Check sheet for the modelled part. Datum: model origin and axes. Units: mm. Face numbers are marked on the shaded views. A direction names the side the tool comes from. Coordinates: 2 decimals unless noted, no trailing zeros. Loops run counter-clockwise (first coordinate to the right, second up) from the corner with the lowest first, then second, coordinate; pieces in that order, holes last.
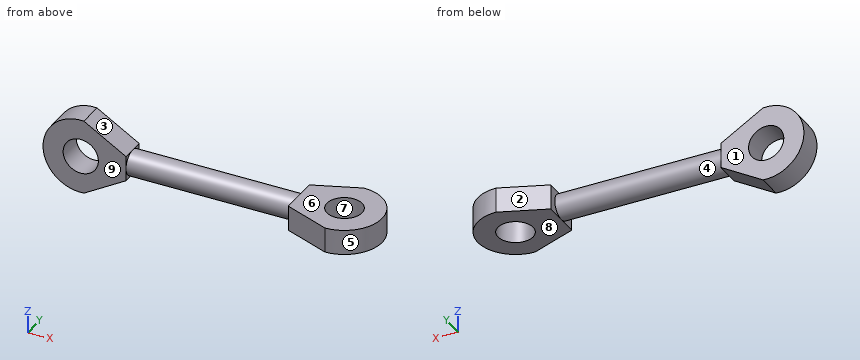
```python
from build123d import *

# Parameters (mm, degrees)
BOSS_EXTRUDE2_DEPTH = 2.5
SKETCH4_R           = 2.5
BOSS_EXTRUDE3_DEPTH = 33.000000000000014
SKETCH8_R           = 3.5000000000000004
BOSS_EXTRUDE4_DEPTH = 2.5


with BuildPart() as part:
    # Sketch1 → Boss-Extrude2 (new, symmetric)
    with BuildSketch(Plane.XY):
        with BuildLine():
            ThreePointArc((7.5, -3.5307e-13), (5.303300858899232, 5.303300858898982), (1.36e-15, 7.500000000000001))
            Line((0, 7.5), (-9.088423691387959, 4))
            Line((-9.088423691387959, 4), (-9.088423691387959, 0))
            Line((-9.088423691387959, 0), (-3.5, 0))
            ThreePointArc((-3.5, 4.3e-16), (2.1e-16, 3.5), (3.5, 0))
            Line((3.5, 0), (7.5, 0))
        make_face()
        with BuildLine():
            ThreePointArc((0, -7.499999999999999), (5.303300858898981, -5.303300858899231), (7.5, -3.5307e-13))
            Line((7.5, 0), (3.5, 0))
            ThreePointArc((3.5, -8.6e-16), (-6.4e-16, -3.5), (-3.5, 4.3e-16))
            Line((-3.5, 0), (-9.088423691387959, 0))
            Line((-9.088423691387959, 0), (-9.088423691387959, -4))
            Line((-9.088423691387959, -4), (0, -7.5))
        make_face()
    extrude(amount=BOSS_EXTRUDE2_DEPTH, both=True)

    # Sketch4 → Boss-Extrude3 (add)
    with BuildSketch(Plane.ZY.offset(9.088423691387959)):
        Circle(SKETCH4_R)
    extrude(amount=BOSS_EXTRUDE3_DEPTH)

    # Sketch8 → Boss-Extrude4 (add, symmetric)
    with BuildSketch(Plane(origin=(0, 0, 0), x_dir=(1, 0, 0), z_dir=(0, 1, 0))):
        with BuildLine():
            Line((-42.08842369138797, 2.5), (-42.08842369138797, -2.5))
            Line((-42.08842369138797, -2.5), (-50.46269365807758, -7.4738518800825435))
            ThreePointArc((-50.46269365807758, -7.4738518800825435), (-58.588423691387945, 9.2e-16), (-50.46269365807758, 7.473851880082519))
            Line((-50.46269365807758, 7.473851880082519), (-42.08842369138797, 2.5))
        make_face()
        with Locations(Location((-51.08842369138797, 0, 0), (0, 0, 270))):
            Circle(SKETCH8_R, mode=Mode.SUBTRACT)
    extrude(amount=BOSS_EXTRUDE4_DEPTH, both=True)


solid = part.part
```
1) Section check A-A on z = 1.5. Enter the section's corners in (x, y).
Answer sheet:
outline: (-58.44, -2.5) - (-54.25, -2.5) - (-54.25, 2.5) - (-58.44, 2.5) - close; (-47.93, -2.5) - (-42.09, -2.5) - (-42.09, -2) - (-9.09, -2) - (-9.09, -4) - (0, -7.5) arc R7.5 ccw to (0, 7.5) - (-9.09, 4) - (-9.09, 2) - (-42.09, 2) - (-42.09, 2.5) - (-47.93, 2.5) - close; hole circle Ø7 at (0, 0)
2) Depth check by flat-ended pin: pin 1 (1.2 mm diameter, centred on y = 1.5, z = -1.5, fed in from +X); pin 2 (4 mm diameter, centred on x = -23.5, y = 3, fed in from -Z); pin 3 (2 mm diameter, centred on y = -3, z = 2, fed in from +X). Enter the tip coordinate at first touch or a pass-through.
Answer sheet:
pin 1: stops at x = 7.45
pin 2: stops at z = -2.29
pin 3: stops at x = 7.23
3) Section check D-D on z = -4.5. Enter the section's corners in (x, y), plus the area to 3 significant figures.
Answer sheet:
outline: (-57.09, -2.5) - (-45.46, -2.5) - (-45.46, 2.5) - (-57.09, 2.5) - close
area: 58.2 mm2
4) Section check C-C on x = -11.5. Enter the section's corners in (y, z).
Answer sheet:
outline: circle Ø5 at (0, 0)
5) Section check B-B on y = 0.75. Enter the section's corners in (x, z), plus the area to 3 significant figures.
Answer sheet:
outline: (-50.46, -7.47) - (-42.09, -2.5) - (-42.09, -2.38) - (-9.09, -2.38) - (-9.09, -2.5) - (-3.42, -2.5) - (-3.42, 2.5) - (-9.09, 2.5) - (-9.09, 2.38) - (-42.09, 2.38) - (-42.09, 2.5) - (-50.46, 7.47) arc R7.5 ccw (long way) to start; (3.42, -2.5) - (7.46, -2.5) - (7.46, 2.5) - (3.42, 2.5) - close; hole circle Ø7 at (-51.09, 0)
area: 349 mm2
6) Scan lines: line 1 (X direction, y = -1.45, z = 0); line 2 (X direction, y = -0.95, z = 0); line 3 (Z direction, x = -3.5, y = -1.5). Record each from-to range of solid material in increasing order.
Answer sheet:
line 1: x = -58.59 to -54.59, -47.59 to -3.19, 3.19 to 7.36
line 2: x = -58.59 to -54.59, -47.59 to -3.37, 3.37 to 7.44
line 3: z = -2.5 to 2.5
7) Set-up check for the marked faces 5, 6, 7, 8 and 9: record each of +Z, -Z, +X, -X, +Y, -Y from which the full face is reachable in a straight line by a thin tool's end or side.
Answer sheet:
face 5: +Z, -Z, +X
face 6: +Z, +X, +Y, -Y
face 7: +Z, -Z
face 8: -Z, +X, +Y, -Y
face 9: +Z, -Z, -X, -Y
8) Mould release check, pull along X, two halves, no side actions. Record for the marked faces 1, 2, 3 and 4: +X half, -X half, draft (parallel to the pull), parting line (faces both ways), or undercut.
Answer sheet:
face 1: draft
face 2: -X half
face 3: +X half
face 4: undercut
